```python
from build123d import *

# Parameters (mm, degrees)
CUT_EXTRUDE1_DEPTH      = 56.524769248
CUT_EXTRUDE1_DEPTH_BACK = 56.524769248
SKETCH2_W               = 36
SKETCH2_H               = 15


with BuildPart() as part:
    # Sketch1 → Revolve1 (revolve)
    with BuildSketch(Plane.XY, mode=Mode.PRIVATE) as revolve1_sk:
        with BuildLine():
            Line((8.808297686, 15.060389461), (8.244359234, 13.670434993))
            Line((8.244359234, 13.670434993), (16.137360004, -5))
            Line((16.137360004, -5), (18, -5))
            Line((18, -5), (18, 35))
            Line((18, 35), (23, 35))
            Line((23, 35), (23, 45))
            Line((23, 45), (18, 45))
            Line((18, 45), (0, 45))
            Line((0, 45), (0, 35.967908311))
            Line((0, 35.967908311), (8.808297686, 35.967908311))
            Line((8.808297686, 35.967908311), (8.808297686, 25.967908311))
            ThreePointArc((8.808297686, 25.967908311), (10.36, 20.514148886), (8.808297686, 15.060389461))
        make_face()
    revolve(revolve1_sk.sketch.rotate(Axis((0, 0, 0), (0, 1, 0)), 90), axis=Axis((0, 0, 0), (0, 1, 0)))

    # Sketch2 → Cut-Extrude1 (cut, two sides: drawn at the far end of the back side and taken through both)
    with BuildSketch(Plane(origin=(0, 0, 0), x_dir=(0, 0, -1), z_dir=(1, 0, 0)).offset(-CUT_EXTRUDE1_DEPTH_BACK)):
        with Locations((0, 2.5)):
            Rectangle(SKETCH2_W, SKETCH2_H)
    extrude(amount=CUT_EXTRUDE1_DEPTH + CUT_EXTRUDE1_DEPTH_BACK, mode=Mode.SUBTRACT)


solid = part.part
```
Can you work these out from the model? Positions are in its coordinate system, mm. A direction names the side the tool comes from. Give positions to 0.01 mm unless a question says otherwise; leave off trailing zeros. Write each loop counter-clockwise with the first axis right and the second up, starting at its lowest first coordinate (ties: lowest second). Pieces come first, ordered by that corner, then holes. Notation, with made-up numbers: (-36, 28.5) -> (-17, 28.5) arc R6 ccw to (-17, 36.5) -> close; hole circle Ø6 at (-3.75, -39.5). An arc over 180 degrees is marked (long way). One line per item, written item: value.
Q1. Imagine slicing it at B-B on x = 0. Please give me the cut outline in (y, z), and give its area (3 significant figures).
Results found:
outline: (10, -18) -> (35, -18) -> (35, -23) -> (45, -23) -> (45, 23) -> (35, 23) -> (35, 18) -> (10, 18) -> (10, 9.8) -> (13.67, 8.24) -> (15.06, 8.81) arc R10.36 cw to (25.97, 8.81) -> (35.97, 8.81) -> (35.97, -8.81) -> (25.97, -8.81) arc R10.36 cw to (15.06, -8.81) -> (13.67, -8.24) -> (10, -9.8) -> close
area: 879 mm^2
Q2. Imagine slicing it at A-A on y = 30. Please give me the cut outline in (x, z).
Results found:
outline: circle Ø36 at (0, 0); hole circle Ø17.62 at (0, 0)
Q3. Imagine slicing it at C-C on z = -14.5. Please give me the cut outline in (x, y).
Results found:
outline: (-17.85, 35) -> (-10.67, 35) -> (-10.67, 10) -> (10.67, 10) -> (10.67, 35) -> (17.85, 35) -> (17.85, 45) -> (-17.85, 45) -> close
Q4. For P1, Ø1, axis at x = 12, z = 18, coming from the -Y side; P2, Ø6, axis at x = 8.5, y = 21.5, coming from the -Z side; P3, Ø14, axis at x = -1.5, z = 3.5, coming from the -Y side; P4, Ø6, axis at x = -1.5, y = 13.5, coming from the +Z side, each with a flat end and sliding along its axis, tell me the tip position at first contact or that it passes through.
Results found:
P1: stops at y = 35
P2: stops at z = -17.14
P3: stops at y = 10
P4: stops at z = 18
Q5. We'd pull the mould along X, two halves only. Please class faces 1 (the face through (-12.165, 22.675, 13.267)), 2 (the face through (8, 10, -8)), 3 (the face through (-2.506, 13.441, -7.956)): +X half, -X half, draft (parallel to the pull), parting line (faces both ways), or undercut.
Results found:
face 1: parting line
face 2: draft
face 3: undercut
Q6. Imagine slicing it at D-D on y = 37. Please give me the cut outline in (x, z).
Results found:
outline: circle Ø46 at (0, 0)
Q7. Please list where these lines run through material, in increasing order: line 1 (X direction, y = 28.5, z = 0); line 2 (Y direction, x = -18.5, z = -8.5); line 3 (Z direction, x = -1, y = 35.5). Write a range as [from, to].
Results found:
line 1: x = [-18, -8.81], [8.81, 18]
line 2: y = [35, 45]
line 3: z = [-22.98, -8.75], [8.75, 22.98]
Q8. Which directions (+Z, -Z, +X, -X, +Y, -Y) give clear straight access to the entire face, cutting with the end or side of a thin tool? Please do faces 4 (the face through (0, 45, 0)), 5 (the face through (12, 35, -14)), 6 (the face through (8.6, 30.9, 1.9)).
Results found:
face 4: +Z, -Z, +X, -X, +Y
face 5: -Y
face 6: none
